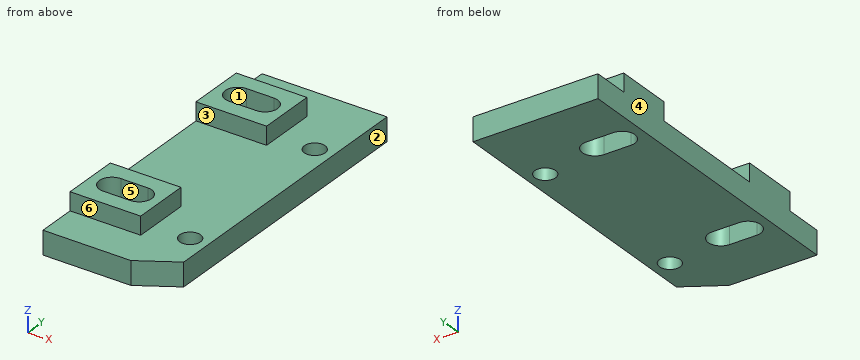
```python
from build123d import *

# Parameters (mm, degrees)
OPPOSITE_END_CROSSBAR_WITH_TWO_ADJUS_2_R       = 1.15
OPPOSITE_END_CROSSBAR_WITH_TWO_ADJUSTABL_DEPTH = 2.6
TWO_START                                      = 2.6
TWO_RAISED_PCB_BOLT_PADS_PROFILE_W             = 7.8
TWO_RAISED_PCB_BOLT_PADS_PROFILE_H             = 6.4
TWO_RAISED_PCB_BOLT_PADS_DEPTH                 = 2


with BuildPart() as part:
    # Opposite end crossbar with two adjus 2 → Opposite end crossbar with two adjustabl (new body)
    with BuildSketch(Plane.XY):
        Polygon((25, -24), (34.7, -24), (38.8, -21.5), (38.8, 10.8), (25, 10.8), align=None)
        with Locations((36.8, -17.6)):
            Circle(OPPOSITE_END_CROSSBAR_WITH_TWO_ADJUS_2_R, mode=Mode.SUBTRACT)
        with Locations((36.8, 2.2)):
            Circle(OPPOSITE_END_CROSSBAR_WITH_TWO_ADJUS_2_R, mode=Mode.SUBTRACT)
        with BuildLine():
            Line((27.4, -17.9), (30.4, -17.9))
            ThreePointArc((30.4, -17.9), (31.8, -16.5), (30.4, -15.1))
            Line((30.4, -15.1), (27.4, -15.1))
            ThreePointArc((27.4, -15.1), (26, -16.5), (27.4, -17.9))
        make_face(mode=Mode.SUBTRACT)
        with BuildLine():
            Line((27.4, 2.1), (30.4, 2.1))
            ThreePointArc((30.4, 2.1), (31.8, 3.5), (30.4, 4.9))
            Line((30.4, 4.9), (27.4, 4.9))
            ThreePointArc((27.4, 4.9), (26, 3.5), (27.4, 2.1))
        make_face(mode=Mode.SUBTRACT)
    extrude(amount=OPPOSITE_END_CROSSBAR_WITH_TWO_ADJUSTABL_DEPTH)

    # Two raised PCB bolt pads profile → Two raised PCB bolt pads (add)
    # profile 1 of 2: a face of its own
    with BuildSketch(Plane.XY.offset(TWO_START)):
        with Locations((28.9, -16.5)):
            Rectangle(TWO_RAISED_PCB_BOLT_PADS_PROFILE_W, TWO_RAISED_PCB_BOLT_PADS_PROFILE_H)
        with BuildLine():
            Line((27.4, -17.9), (30.4, -17.9))
            ThreePointArc((30.4, -17.9), (31.8, -16.5), (30.4, -15.1))
            Line((30.4, -15.1), (27.4, -15.1))
            ThreePointArc((27.4, -15.1), (26, -16.5), (27.4, -17.9))
        make_face(mode=Mode.SUBTRACT)
    # profile 2 of 2: a face of its own
    with BuildSketch(Plane.XY.offset(TWO_START)):
        with Locations((28.9, 3.5)):
            Rectangle(TWO_RAISED_PCB_BOLT_PADS_PROFILE_W, TWO_RAISED_PCB_BOLT_PADS_PROFILE_H)
        with BuildLine():
            Line((27.4, 2.1), (30.4, 2.1))
            ThreePointArc((30.4, 2.1), (31.8, 3.5), (30.4, 4.9))
            Line((30.4, 4.9), (27.4, 4.9))
            ThreePointArc((27.4, 4.9), (26, 3.5), (27.4, 2.1))
        make_face(mode=Mode.SUBTRACT)
    extrude(amount=TWO_RAISED_PCB_BOLT_PADS_DEPTH)


solid = part.part
```
Model file for the job. Use its own axes, mm. Face numbers are marked on the shaded views. A direction names the side the tool comes from. Give positions to 0.01 mm unless a question says otherwise; leave off trailing zeros. Write each loop counter-clockwise with the first axis right and the second up, starting at its lowest first coordinate (ties: lowest second). Pieces come first, ordered by that corner, then holes. Notation, with made-up numbers: M 34,4.25 L 54,4.25 A17 ccw 54,30.25 Z; hole C -15.5,27 d10. An arc over 180 degrees is marked long. Use a Markdown table: item, result.
1) Tool access for the marked faces 1, 2 and 3: list every direction of +Z, -Z, +X, -X, +Y, -Y with a clear straight run to the whole face (end or side of a thin tool).
Responses:
| item | result |
|---|---|
| face 1 | +Z, -Z |
| face 2 | +Z, -Z, +X, +Y, -Y |
| face 3 | +Z, +X, -X |
2) Pin check, flat tips, straight feed: pin 1 (1.6 mm diameter, centred on x = 28.5, z = 4, fed in from +Y); pin 2 (1 mm diameter, centred on x = 27.5, z = 3.5, fed in from -Y). Stop position of each tip, or through.
Responses:
| item | result |
|---|---|
| pin 1 | stops at y = 6.7 |
| pin 2 | stops at y = -19.7 |
3) Drill centre lines: line 1 (Y direction, x = 29, z = 2.25); line 2 (Y direction, x = 36.8, z = 1.4); line 3 (Y direction, x = 31.25, z = 2.9). Where is each one in solid material? Low to high. Write a range as from..to.
Responses:
| item | result |
|---|---|
| line 1 | y = -24..-17.9, -15.1..2.1, 4.9..10.8 |
| line 2 | y = -22.72..-18.75, -16.45..1.05, 3.35..10.8 |
| line 3 | y = -19.7..-17.61, -15.39..-13.3, 0.3..2.39, 4.61..6.7 |
4) Pull direction Y, two halves, no side cores. Call the marked faces 4, 5 and 6: +Y half, -Y half, draft (parallel to the pull), parting line (faces both ways), or undercut.
Responses:
| item | result |
|---|---|
| face 4 | draft |
| face 5 | undercut |
| face 6 | -Y half |
5) Cut at D-D (y = -9). List the corners of the cut face in (x, z), and give its area (3 significant figures).
Responses:
| item | result |
|---|---|
| outline | M 25,0 L 38.8,0 L 38.8,2.6 L 25,2.6 Z |
| area | 35.9 mm2 |
6) Cut at B-B (x = 28.25). List the corners of the cut face in (y, z).
Responses:
| item | result |
|---|---|
| outline | M -24,0 L -17.9,0 L -17.9,4.6 L -19.7,4.6 L -19.7,2.6 L -24,2.6 Z; M -15.1,0 L 2.1,0 L 2.1,4.6 L 0.3,4.6 L 0.3,2.6 L -13.3,2.6 L -13.3,4.6 L -15.1,4.6 Z; M 4.9,0 L 10.8,0 L 10.8,2.6 L 6.7,2.6 L 6.7,4.6 L 4.9,4.6 Z |
7) Cut at A-A (z = 3.2). List the corners of the cut face in (x, y), and give its area (3 significant figures).
Responses:
| item | result |
|---|---|
| outline | M 25,-19.7 L 32.8,-19.7 L 32.8,-13.3 L 25,-13.3 Z; M 25,0.3 L 32.8,0.3 L 32.8,6.7 L 25,6.7 Z; hole M 27.4,-17.9 L 30.4,-17.9 A1.4 ccw 30.4,-15.1 L 27.4,-15.1 A1.4 ccw Z; hole M 27.4,2.1 L 30.4,2.1 A1.4 ccw 30.4,4.9 L 27.4,4.9 A1.4 ccw Z |
| area | 70.7 mm2 |
8) Cut at C-C (y = 3). List the corners of the cut face in (x, z), and give its area (3 significant figures).
Responses:
| item | result |
|---|---|
| outline | M 25,0 L 26.09,0 L 26.09,4.6 L 25,4.6 Z; M 31.71,0 L 35.97,0 L 35.97,2.6 L 32.8,2.6 L 32.8,4.6 L 31.71,4.6 Z; M 37.63,0 L 38.8,0 L 38.8,2.6 L 37.63,2.6 Z |
| area | 21.4 mm2 |
